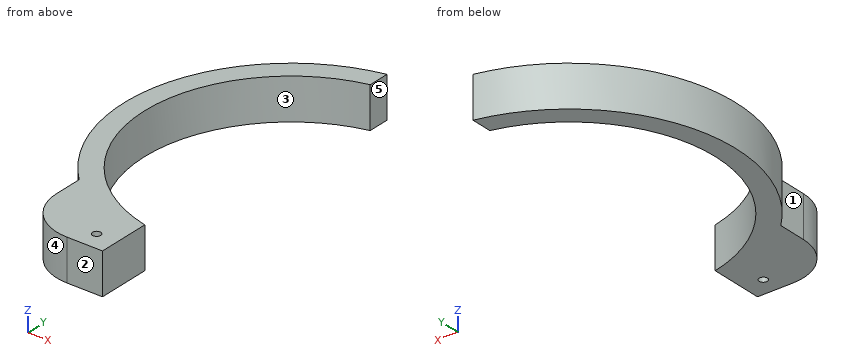
```python
from build123d import *

# Parameters (mm, degrees)
SKETCH1_R           = 1
BOSS_EXTRUDE1_DEPTH = 10
SKETCH2_W           = 8.204002356
SKETCH2_H           = 9.353246275
CUT_EXTRUDE1_DEPTH  = 10


with BuildPart() as part:
    # Sketch1 → Boss-Extrude1 (new body)
    with BuildSketch(Plane.XY):
        with BuildLine():
            ThreePointArc((-8, -34.586847211), (-35.270973023, 4.025973423), (0, 35.5))
            Line((0, 35.5), (0, 40.5))
            ThreePointArc((0, 40.5), (-37.417121067, 15.498679011), (-28.637824638, -28.637824638))
            Line((-28.637824638, -28.637824638), (-28.637824638, -35.5))
            ThreePointArc((-28.637824638, -35.5), (-25.123106012, -43.985281374), (-16.637824638, -47.5))
            Line((-16.637824638, -47.5), (-8, -47.5))
            Line((-8, -47.5), (-8, -34.586847211))
        make_face()
        with Locations((-13, -42.999876828)):
            Circle(SKETCH1_R, mode=Mode.SUBTRACT)
    extrude(amount=BOSS_EXTRUDE1_DEPTH)

    # Sketch2 → Cut-Extrude1 (cut)
    with BuildSketch(Plane.XY.offset(10)):
        with Locations((-4.102001178, 35.823376862)):
            Rectangle(SKETCH2_W, SKETCH2_H)
    extrude(amount=-CUT_EXTRUDE1_DEPTH, mode=Mode.SUBTRACT)


solid = part.part
```
Source: CAD feature listing. Evaluate the final solid. Frame: model axes, mm. Face numbers are marked on the shaded views. A direction names the side the tool comes from. Give positions to 0.01 mm unless a question says otherwise; leave off trailing zeros. Order: outer loops, then holes, each group sorted by start corner. A loop starts at its lowest first (then second) coordinate and runs counter-clockwise, first axis right, second up. Notation, with made-up numbers: (82, -38.75) -> (112, -38.75) arc R32 cw to (112, -9.75) -> close; hole circle Ø2 at (15.25, -16). An arc over 180 degrees is marked (long way). Use a Markdown table: item, result.
Q1. First-contact query: P1, Ø3, axis at y = 24.5, z = 7, coming from the +X side; P2, Ø1.6, axis at x = -13, y = -43, coming from the -Z side; P3, Ø6, axis at x = -12, z = 1, coming from the +Y side; P4, Ø1.5, axis at y = 36.5, z = 7, coming from the +X side. Flat tips, straight axial feed; report the tip coordinate or a pass-through.
A:
| item | result |
|---|---|
| P1 | x = -24.17 |
| P2 | through |
| P3 | y = 39.49 |
| P4 | x = -8.2 |
Q2. Section C-C (x = -13). Return the cut outline in (y, z), and give its area (3 significant figures).
A:
| item | result |
|---|---|
| outline | (-47.5, 0) -> (-44, 0) -> (-44, 10) -> (-47.5, 10) -> close; (-42, 0) -> (-33.03, 0) -> (-33.03, 10) -> (-42, 10) -> close; (33.03, 0) -> (38.36, 0) -> (38.36, 10) -> (33.03, 10) -> close |
| area | 178 mm^2 |
Q3. Section B-B (z = 5.5). Return the cut outline in (x, y), and give its area (3 significant figures).
A:
| item | result |
|---|---|
| outline | (-28.64, -35.5) arc R12 ccw to (-16.64, -47.5) -> (-8, -47.5) -> (-8, -34.59) arc R35.5 cw to (-8.2, 34.54) -> (-8.2, 39.66) arc R40.5 ccw to (-28.64, -28.64) -> close; hole circle Ø2 at (-13, -43) |
| area | 729 mm^2 |
Q4. Section D-D (y = 16). Return the cut outline in (x, z).
A:
| item | result |
|---|---|
| outline | (-37.21, 0) -> (-31.69, 0) -> (-31.69, 10) -> (-37.21, 10) -> close |
Q5. Material intervals for line 1 (Y direction, x = -13, z = 3.5); line 2 (Y direction, x = -24, z = 7.5); line 3 (Y direction, x = -31.5, z = 7.25), sorted ascending. Write a range as [from, to].
A:
| item | result |
|---|---|
| line 1 | [-47.5, -44], [-42, -33.03], [33.03, 38.36] |
| line 2 | [-44.98, -26.16], [26.16, 32.62] |
| line 3 | [-25.46, -16.37], [16.37, 25.46] |
Q6. Section A-A (x = -24). Return the cut outline in (y, z), and give its area (3 significant figures).
A:
| item | result |
|---|---|
| outline | (-44.98, 0) -> (-26.16, 0) -> (-26.16, 10) -> (-44.98, 10) -> close; (26.16, 0) -> (32.62, 0) -> (32.62, 10) -> (26.16, 10) -> close |
| area | 253 mm^2 |
Q7. Pull-direction query (Y, two-part tool) for the marked faces 3, 4 and 5; classes: +Y half, -Y half, draft (parallel to the pull), parting line (faces both ways), or undercut.
A:
| item | result |
|---|---|
| face 3 | undercut |
| face 4 | -Y half |
| face 5 | draft |
Q8. Access query for the marked faces 1 and 2. Directions: +Z, -Z, +X, -X, +Y, -Y. A direction counts if a zero-diameter tool reaches every point of the face in a straight line with its end or side. Return the directions, or none.
A:
| item | result |
|---|---|
| face 1 | +Z, -Z, -X, -Y |
| face 2 | +Z, -Z, +X, -X, -Y |
